from build123d import *

# Parameters (mm, degrees)
F0_W        = 65
F0_H        = 65
F0_R        = 8.5
F1_DEPTH    = 75
F2_T        = -1.778
F3_T1_DEPTH = 61.444
F3_T3_DEPTH = 61.444


# Not quite as in the source:
# - a fillet or chamfer that OpenCascade refuses, or shapes differently, is made with other operations: its cross-section is extruded or revolved along the edge and cut away or added


with BuildPart() as f1:
    # F0 (on Top) → F1 (new body)
    with BuildSketch(Plane.XY):
        Rectangle(F0_W, F0_H)
        with Locations((-16.25, -16.25)):
            Circle(F0_R, mode=Mode.SUBTRACT)
        with Locations((16.25, -16.25)):
            Circle(F0_R, mode=Mode.SUBTRACT)
        with Locations((-16.25, 16.25)):
            Circle(F0_R, mode=Mode.SUBTRACT)
        with Locations((16.25, 16.25)):
            Circle(F0_R, mode=Mode.SUBTRACT)
    extrude(amount=F1_DEPTH)

    # F2
    f2_openings = [f1.faces().sort_by_distance(p)[0] for p in [
        (0, 0, 0),
    ]]
    offset(amount=F2_T, openings=f2_openings)

    # F3: fillet of radius 5.08 on 8 edges, made by hand

    # F3_s2 → F3_t1 (join)
    with BuildSketch(Plane.YZ.offset(-30.722)):
        with BuildLine():
            ThreePointArc((30.722, 68.142), (29.2341024484, 71.7341024484), (25.642, 73.222))
            Line((25.642, 73.222), (30.722, 73.222))
            Line((30.722, 73.222), (30.722, 68.142))
        make_face()
        with BuildLine():
            ThreePointArc((-30.722, 68.142), (-29.2341024484, 71.7341024484), (-25.642, 73.222))
            Line((-25.642, 73.222), (-30.722, 73.222))
            Line((-30.722, 73.222), (-30.722, 68.142))
        make_face()
    extrude(amount=F3_T1_DEPTH)

    # F3_s4 → F3_t3 (join)
    with BuildSketch(Plane.XZ.offset(-30.722)):
        with BuildLine():
            ThreePointArc((-30.722, 68.142), (-29.2341024484, 71.7341024484), (-25.642, 73.222))
            Line((-25.642, 73.222), (-30.722, 73.222))
            Line((-30.722, 73.222), (-30.722, 68.142))
        make_face()
        with BuildLine():
            ThreePointArc((30.722, 68.142), (29.2341024484, 71.7341024484), (25.642, 73.222))
            Line((25.642, 73.222), (30.722, 73.222))
            Line((30.722, 73.222), (30.722, 68.142))
        make_face()
    extrude(amount=F3_T3_DEPTH)

    # F3_s5 → F3_t6 (revolve)
    with BuildSketch(Plane.XZ.offset(16.25)):
        with BuildLine():
            ThreePointArc((-0.892, 73.222), (-4.4841024484, 71.7341024484), (-5.972, 68.142))
            Line((-5.972, 68.142), (-5.972, 73.222))
            Line((-5.972, 73.222), (-0.892, 73.222))
        make_face()
    revolve(axis=Axis((-16.25, -16.25, 73.222), (0, 0, -1)))

    # F3_s7 → F3_t8 (revolve)
    with BuildSketch(Plane.XZ.offset(16.25)):
        with BuildLine():
            ThreePointArc((31.608, 73.222), (28.0158975516, 71.7341024484), (26.528, 68.142))
            Line((26.528, 68.142), (26.528, 73.222))
            Line((26.528, 73.222), (31.608, 73.222))
        make_face()
    revolve(axis=Axis((16.25, -16.25, 73.222), (0, 0, -1)))

    # F3_s9 → F3_t10 (revolve)
    with BuildSketch(Plane.XZ.offset(-16.25)):
        with BuildLine():
            ThreePointArc((-0.892, 73.222), (-4.4841024484, 71.7341024484), (-5.972, 68.142))
            Line((-5.972, 68.142), (-5.972, 73.222))
            Line((-5.972, 73.222), (-0.892, 73.222))
        make_face()
    revolve(axis=Axis((-16.25, 16.25, 73.222), (0, 0, -1)))

    # F3_s11 → F3_t12 (revolve)
    with BuildSketch(Plane.XZ.offset(-16.25)):
        with BuildLine():
            ThreePointArc((31.608, 73.222), (28.0158975516, 71.7341024484), (26.528, 68.142))
            Line((26.528, 68.142), (26.528, 73.222))
            Line((26.528, 73.222), (31.608, 73.222))
        make_face()
    revolve(axis=Axis((16.25, 16.25, 73.222), (0, 0, -1)))


solid = f1.part
Source: CAD feature listing. Evaluate the final solid. Frame: model axes, mm. A direction names the side the tool comes from. Round coordinates to 2 decimals unless told otherwise and drop trailing zeros. Loops run counter-clockwise (first coordinate to the right, second up) from the corner with the lowest first, then second, coordinate; pieces in that order, holes last. Notation, with made-up numbers: M 60.25,-19.75 L 80.25,-19.75 A23 cw 80.25,1.25 Z; hole C 30,83 d9. An arc over 180 degrees is marked long. Return JSON: item names as keys, results as strings. Group by question number.
1. Material intervals for line 1 along Y through (x, z) = (-16.25, 50.5); line 2 along X through (y, z) = (-16, 22); line 3 along Y through (x, z) = (3, 46), sorted ascending. Write a range as from..to.
2. Pin query (flat end, axial travel): pin 1 (15.5 mm diameter, centred on x = -16.25, y = 16.25, fed in from -Z). Return the tip coordinate at first contact, or that it passes through.
3. Section query A-A on z = 57.5. State how many separate pieces and enclosed holes the cut face has, and give its area (3 significant figures).
4. Section query B-B on y = 16.25. Output: boundary loops of the cut face in (x, z) (3 decimals), and give its area (3 significant figures).
5. Reachability of faces 1 (the face through (0, 0, 75)), 2 (the face through (-26.52, -15.8, 33.59)) from +Z, -Z, +X, -X, +Y, -Y: full face, straight path, thin tool, end or side. Return the list, or none.
6. Mould query, pull axis X, two halves, no side actions, for faces 3 (the face through (29.835, 0.43, 71.01)), 4 (the face through (32.5, 0, 37)), 5 (the face through (12, 24, 0)), 6 (the face through (-0.43, -29.835, 71.01)). Classes: released by +X, released by -X, zero draft, split by the parting line, or undercut.
Checks:
{
 "1": {"line 1": "y = -32.5..-30.72, -26.53..-24.75, -7.75..-5.97, 5.97..7.75, 24.75..26.53, 30.72..32.5", "line 2": "x = -32.5..-30.72, -26.52..-24.75, -7.75..-5.98, 5.98..7.75, 24.75..26.52, 30.72..32.5", "line 3": "y = -32.5..-30.72, 30.72..32.5"},
 "2": {"pin 1": "passes through"},
 "3": {"separate pieces": "5", "enclosed holes": "5", "area": "869 mm²"},
 "4": {"outline": "M -32.5,0 L -30.722,0 L -30.722,68.142 A5.08 cw -28.625,72.254 A5.08 cw -26.528,68.142 L -26.528,0 L -24.75,0 L -24.75,75 L -32.5,75 Z; M -7.75,0 L -5.972,0 L -5.972,68.142 A5.08 cw -0.892,73.222 L 0.892,73.222 A5.08 cw 5.972,68.142 L 5.972,0 L 7.75,0 L 7.75,75 L -7.75,75 Z; M 24.75,0 L 26.528,0 L 26.528,68.142 A5.08 cw 28.625,72.254 A5.08 cw 30.722,68.142 L 30.722,0 L 32.5,0 L 32.5,75 L 24.75,75 Z", "area": "866 mm²"},
 "5": {"face 1": "+Z, +X, -X, +Y, -Y", "face 2": "-Z"},
 "6": {"face 3": "undercut", "face 4": "released by +X", "face 5": "zero draft", "face 6": "undercut"}
}
